```python
from build123d import *

# Parameters (mm, degrees)
F1_DEPTH = 25.4
F2_W     = 19.62
F2_H     = 19.62
F3_DEPTH = 25
F4_DEPTH = 25


with BuildPart() as f1:
    # F0 (on Front) → F1 (new body)
    with BuildSketch(Plane.XZ):
        Polygon((36.31416, 28.91813), (-21.683757, 28.426622), (-21.683757, -10.573378), (16.316243, -10.573378), (16.316243, 8.91813), (36.31416, 8.91813), align=None)
    extrude(amount=F1_DEPTH)

    # F2 (on Front) → F3 (join)
    with BuildSketch(Plane.XZ):
        with Locations((-11.983198, -0.2484)):
            Rectangle(F2_W, F2_H)
    extrude(amount=-F3_DEPTH)

    # F2 (on Front) → F4 (join)
    with BuildSketch(Plane.XZ):
        with Locations((-11.983198, -0.2484)):
            Rectangle(F2_W, F2_H)
    extrude(amount=F4_DEPTH)


solid = f1.part
```
CAD build for the part. Positions are in the model's coordinates, mm. A direction names the side the tool comes from. Give positions to 0.01 mm unless a question says otherwise; leave off trailing zeros. Order: outer loops, then holes, each group sorted by start corner. A loop starts at its lowest first (then second) coordinate and runs counter-clockwise, first axis right, second up.
(1) Saw through at B-B, the plane y = -16.5. Give the cut face in (x, z), then the cut area to 3 significant figures.
(2) Saw through at C-C, the plane z = 10.5. Give the cut face in (x, y).
(3) Flat gauge pins, fed straight in: pin 1 (6 mm diameter, centred on y = -20, z = 20, fed in from -X); pin 2 (9.5 mm diameter, centred on y = -9.5, z = -3.5, fed in from +X); pin 3 (12 mm diameter, centred on y = 13.5, z = -5, fed in from +X). Where does each tip first touch, or does it go through?
(4) Saw through at A-A, the plane x = -8. Give the cut face in (y, z).
(5) Drill centre lines: L1, parallel to Y at x = 12, z = 14.5; L2, parallel to X at y = -3, z = 18.5; L3, parallel to X at y = -15, z = 5. Where is each one in solid material? Low to high.
(6) Tool access for faces 1 (the flat face through (-12, 25, 0)), 2 (the flat face through (16.316, -13, -1)), 3 (the flat face through (-2.173, 12, 0)): list every direction of +Z, -Z, +X, -X, +Y, -Y with a clear straight run to the whole face (end or side of a thin tool).
(7) Saw through at D-D, the plane y = 13. Give the cut face in (x, z), then the cut area to 3 significant figures.
Results found:
1. outline: (-21.79, -10.06) - (-21.68, -10.06) - (-21.68, -10.57) - (16.32, -10.57) - (16.32, 8.92) - (36.31, 8.92) - (36.31, 28.92) - (-21.68, 28.43) - (-21.68, 9.56) - (-21.79, 9.56) - close
1. area: 1,890 mm2
2. outline: (-21.68, -25.4) - (36.31, -25.4) - (36.31, 0) - (-21.68, 0) - close
3. pin 1: stops at x = -21.68
3. pin 2: stops at x = 16.32
3. pin 3: stops at x = -2.17
4. outline: (-25.4, -10.57) - (0, -10.57) - (0, -10.06) - (25, -10.06) - (25, 9.56) - (0, 9.56) - (0, 28.54) - (-25.4, 28.54) - close
5. L1: y = -25.4 to 0
5. L2: x = -21.68 to 36.31
5. L3: x = -21.79 to 16.32
6. face 1: +Z, -Z, +X, -X, +Y
6. face 2: -Z, +X, +Y, -Y
6. face 3: +Z, -Z, +X, +Y
7. outline: (-21.79, -10.06) - (-2.17, -10.06) - (-2.17, 9.56) - (-21.79, 9.56) - close
7. area: 385 mm2
